Autodesk Inventor part; units mm, degrees
ref_plane "YZ Plane" through (0, 0, 0) normal (1, 0, 0) x (0, 1, 0)
ref_plane "XZ Plane" through (0, 0, 0) normal (0, 1, 0) x (-1, 0, 0)
ref_plane "XY Plane" through (0, 0, 0) normal (0, 0, 1) x (1, 0, 0)
sketch "Szkic1" plane through (0, 0, 0) normal (0, 1, 0) x (-1, 0, 0)
  line L0 (30, -30) -> (-30, -30)
  line L1 (-30, -30) -> (-30, 30)
  line L2 (-30, 30) -> (30, 30)
  line L3 (30, 30) -> (30, -30)
  line L4 (30, -30) -> (-30, 30) construction
  line L5 (-30, -30) -> (30, 30) construction
  point P0 (0, 0)
  dimension "d0" = 60
  dimension "d1" = 60
extrude "Wyciągnięcie proste1" add sketch "Szkic1" along normal blind 3
sketch "Szkic2" plane through (0, 3, 0) normal (0, 1, 0) x (1, 0, 0)
  line L0 (10, -12) -> (-10, -12)
  line L1 (-10, -12) -> (-10, -15)
  line L2 (-10, -15) -> (10, -15)
  line L3 (10, -15) -> (10, -12)
  point P0 (0, 0)
  dimension "d4" = 20
  dimension "d5" = 3
  dimension "d6" = 12
  dimension "d7" = 10
sketch "Szkic3" plane through (0, 3, 0) normal (0, 1, 0) x (1, 0, 0)
  point P0 (0, 0)
sketch "Szkic4" plane through (0, 3, 0) normal (0, 1, 0) x (1, 0, 0)
  line L0 (-13, 17.5) -> (23, 17.5)
  line L1 (23, 17.5) -> (23, 20.5)
  line L2 (23, 20.5) -> (-13, 20.5)
  line L3 (-13, 20.5) -> (-13, 17.5)
  point P0 (0, 0)
  dimension "d8" = 3
  dimension "d9" = 36
  dimension "d10" = 17.5
  dimension "d11" = 13
extrude "Wyciągnięcie proste2" add sketch "Szkic4" along normal blind 30
sketch "Szkic5" plane through (23, 3, -20.5) normal (0, 0, -1) x (-1, 0, 0)
  line L0 (0, 30) -> (36, 30)
  line L1 (36, 0) -> (36, 30)
  arc A0 (17.4615, 14.6923) -> (17.4615, 19.3077) centre (23, 17) ccw
  arc A1 (17.4615, 19.3077) -> (17.4615, 14.6923) centre (16.5, 17) ccw
  line L2 (0, 0) -> (0, 30)
  circle A2 centre (4.5, 17) radius 1.25
  circle A3 centre (31.5, 17) radius 1.25
  point P0 (23, -3)
  dimension "d14" = 13
  dimension "d15" = 13
  dimension "d16" = 12
  dimension "d17" = 6.5
  dimension "d18" = 5
  dimension "d19" = 4.5
  dimension "d20" = 4.5
  dimension "d21" = 2.5
  dimension "d22" = 2.5
extrude "Wyciągnięcie proste3" cut sketch "Szkic5" against normal blind 30
sketch "Szkic6" plane through (0, 3, 0) normal (0, 1, 0) x (1, 0, 0)
  point P0 (0, 0)
extrude "Wyciągnięcie proste4" add sketch "Szkic2" along normal blind 30
sketch "Szkic7" plane through (10, 3, 12) normal (0, 0, -1) x (-1, 0, 0)
  point P0 (10, -3)
sketch "Szkic8" plane through (-10, 3, 15) normal (0, 0, 1) x (1, 0, 0)
  line L0 (20, 0) -> (0, 0)
  point P0 (10, -3)
  point P1 (10, 17)
  dimension "d27" = 17
hole "Otwór1" at (0, 20, 15) direction (0, 0, -1) diameter 3.2 end through all
sketch "Szkic9" plane through (-30, 0, -30) normal (-1, 0, 0) x (0, 0, 1)
  line L0 (60, 3) -> (0, 3)
  line L1 (0, 0) -> (60, 0)
  line L2 (60, 0) -> (60, 3)
  line L3 (60, 3) -> (0, 3)
  line L4 (0, 3) -> (0, 0)
  point P0 (30, 0)
extrude "Wyciągnięcie proste5" add sketch "Szkic9" along normal blind 60
sketch "Szkic10" plane through (0, 3, 0) normal (0, 1, 0) x (1, 0, 0)
  line L0 (-13, 20.5) -> (-13, 17.5)
  line L1 (30, -30) -> (-90, -30)
  point P0 (0, 0)
  point P1 (-27, -19)
  point P2 (-27, 8.9)
  point P3 (-77.8, 24)
  point P4 (-79.1, -24.1)
  dimension "d38" = 14
  dimension "d39" = 11
  dimension "d40" = 27.9
  dimension "d41" = 50.8
  dimension "d42" = 54
  dimension "d43" = 1.3
  dimension "d44" = 5.9
hole "Otwór2" at (-27, 3, 19) at (-27, 3, -8.9) at (-77.8, 3, -24) at (-79.1, 3, 24.1) direction (0, -1, 0) diameter 3 end through all
properties part number "podstawa" material "Drewno (brzoza)"
Geometry check sheet. Reference: the model listing, model coordinates, mm. A direction names the side the tool comes from. Give positions to 0.01 mm unless a question says otherwise; leave off trailing zeros. Write each loop counter-clockwise with the first axis right and the second up, starting at its lowest first coordinate (ties: lowest second). Pieces come first, ordered by that corner, then holes. Notation, with made-up numbers: (9, -8.75) - (48, -8.75) arc R19 cw to (48, -2.75) - close; hole circle Ø11 at (48, 33). An arc over 180 degrees is marked (long way). Use a Markdown table: item, result.
Q1. Set-up check for faces 1 (the face through (5, 14, -20.5)), 2 (the face through (0, 18, 15)), 3 (the face through (-13, 18, -19)), 4 (the face through (5, 14, -17.5)), 5 (the face through (10, 18, 14)): record each of +Z, -Z, +X, -X, +Y, -Y from which the full face is reachable in a straight line by a thin tool's end or side.
Computed:
| item | result |
|---|---|
| face 1 | -Z, +X, -X, +Y |
| face 2 | +Z, +X, -X, +Y |
| face 3 | +Z, -Z, -X, +Y |
| face 4 | +X, -X, +Y |
| face 5 | +Z, +X, +Y |
Q2. Section check A-A, the plane z = -24. Enter the section's corners in (x, y).
Computed:
| item | result |
|---|---|
| outline | (-90, 0) - (-79.3, 0) - (-79.3, 3) - (-90, 3) - close; (-76.3, 0) - (30, 0) - (30, 3) - (-76.3, 3) - close |
Q3. Thickness scan on L1, parallel to Y at x = 0, z = -18.25; L2, parallel to X at y = 0.9, z = -24; L3, parallel to Z at x = 3, y = 9. Record the ranges inside material, lowest first. Write a range as [from, to].
Computed:
| item | result |
|---|---|
| L1 | y = [0, 14], [26, 33] |
| L2 | x = [-90, -79.3], [-76.3, 30] |
| L3 | z = [-20.5, -17.5], [12, 15] |
Q4. Section check C-C, the plane x = 0. Enter the section's corners in (y, z).
Computed:
| item | result |
|---|---|
| outline | (0, -30) - (3, -30) - (3, -20.5) - (14, -20.5) - (14, -17.5) - (3, -17.5) - (3, 12) - (18.4, 12) - (18.4, 15) - (3, 15) - (3, 30) - (0, 30) - close; (21.6, 12) - (33, 12) - (33, 15) - (21.6, 15) - close; (26, -20.5) - (33, -20.5) - (33, -17.5) - (26, -17.5) - close |
Q5. Go/stop test with flat-tipped pins: P1, Ø1, axis at y = 26.5, z = -15.5, coming from the -X side; P2, Ø3.5, axis at y = 11, z = 14, coming from the -X side; P3, Ø10, axis at x = -3.5, y = 13, coming from the +Z side; P4, Ø3.5, axis at y = 10.5, z = 14, coming from the +X side. Record where each tip stops, or that it passes through.
Computed:
| item | result |
|---|---|
| P1 | passes through |
| P2 | stops at x = -10 |
| P3 | stops at z = 15 |
| P4 | stops at x = 10 |
Q6. Section check D-D, the plane x = -27. Enter the section's corners in (y, z).
Computed:
| item | result |
|---|---|
| outline | (0, -30) - (3, -30) - (3, -10.4) - (0, -10.4) - close; (0, -7.4) - (3, -7.4) - (3, 17.5) - (0, 17.5) - close; (0, 20.5) - (3, 20.5) - (3, 30) - (0, 30) - close |
Q7. Section check B-B, the plane y = 12. Enter the section's corners in (x, z).
Computed:
| item | result |
|---|---|
| outline | (-13, -20.5) - (23, -20.5) - (23, -17.5) - (-13, -17.5) - close; (-10, 12) - (10, 12) - (10, 15) - (-10, 15) - close |
Q8. Draft check along X on faces 6 (the face through (5, 33, -19)), 7 (the face through (-90, 2, 0)), 8 (the face through (-28.487, 1.479, -9.095)). Enter one of: pulls with the +X half, pulls with the -X half, needs draft (parallel to the pull), parting line crosses it, or undercut.
Computed:
| item | result |
|---|---|
| face 6 | needs draft |
| face 7 | pulls with the -X half |
| face 8 | undercut |
